```python
from build123d import *

# Parameters (mm, degrees)
SALIENTE_EXTRUIR1_DEPTH       = 3
REDONDEO1_R                   = 4
CROQUIS4_R                    = 2
CORTAR_EXTRUIR1_DEPTH         = 10
CROQUIS5_R                    = 2
CORTAR_EXTRUIR2_DEPTH         = 10
TALADRO_ROSCADO_M31_D         = 2.5
TALADRO_ROSCADO_M31_DEPTH     = 8.5
TALADRO_ROSCADO_M31_TIP       = 0.751075774
CROQUIS13_R                   = 2
CORTAR_EXTRUIR6_DEPTH         = 438.724799389
CROQUIS14_R                   = 2
CORTAR_EXTRUIR7_DEPTH         = 438.724799389
CORTAR_EXTRUIR9_DEPTH         = 438.724799389
TALADRO_ROSCADO_M32_D         = 2.5
TALADRO_ROSCADO_M32_DEPTH     = 8.5
TALADRO_ROSCADO_M32_TIP       = 0.751075774
TALADRO_ROSCADO_M33_OUTLINE_R = 1.25
TALADRO_ROSCADO_M33_DEPTH     = 3
CROQUIS22_R                   = 2
CORTAR_EXTRUIR10_DEPTH        = 438.724799389
CROQUIS23_R                   = 2
CORTAR_EXTRUIR11_DEPTH        = 438.724799389
TALADRO_ROSCADO_M34_OUTLINE_R = 1.25
TALADRO_ROSCADO_M34_DEPTH     = 3
CROQUIS26_R                   = 2
CORTAR_EXTRUIR12_DEPTH        = 438.724799389
TALADRO_ROSCADO_M35_OUTLINE_R = 1.25
TALADRO_ROSCADO_M35_DEPTH     = 3
CROQUIS31_R                   = 2
CORTAR_EXTRUIR13_DEPTH        = 438.724799389
CORTAR_EXTRUIR14_DEPTH        = 438.724799389


# Read off the part's stored shape, not the designer's step: Taladro roscado M33, Taladro roscado M34, Taladro roscado M35
with BuildPart() as part:
    # Croquis1 → Saliente-Extruir1 (new body)
    with BuildSketch(Plane(origin=(0, 0, 0), x_dir=(1, 0, 0), z_dir=(0, 1, 0))):
        Polygon((0, 0), (-413, 0), (-413, 45), (-338, 45), (-338, 123), (-190, 123), (-190, 107), (-125, 107), (-125, 145), (-75, 145), (-75, 97), (0, 97), align=None)
    saliente_extruir1 = extrude(amount=SALIENTE_EXTRUIR1_DEPTH)

    # Simetría1: Saliente-Extruir1 across plane
    add(saliente_extruir1.mirror(Plane(origin=(0, 3, 0), x_dir=(1, 0, 0), z_dir=(0, 0, -1))))

    # Redondeo1
    redondeo1_edges = [part.edges().sort_by_distance(p)[0] for p in [
        (-413, 1.5, -45),
        (-338, 1.5, -45),
        (-338, 1.5, -123),
        (-190, 1.5, -123),
        (-190, 1.5, -107),
        (-125, 1.5, -107),
        (-125, 1.5, -145),
        (-75, 1.5, -145),
        (-75, 1.5, -97),
        (0, 1.5, -97),
        (0, 1.5, 97),
        (-413, 1.5, 45),
        (-338, 1.5, 45),
        (-338, 1.5, 123),
        (-190, 1.5, 123),
        (-190, 1.5, 107),
        (-125, 1.5, 107),
        (-125, 1.5, 145),
        (-75, 1.5, 145),
        (-75, 1.5, 97),
    ]]
    fillet(redondeo1_edges, radius=REDONDEO1_R)

    # Croquis4 → Cortar-Extruir1 (cut)
    with BuildSketch(Plane(origin=(0, 3, 0), x_dir=(1, 0, 0), z_dir=(0, 1, 0))):
        with Locations(Location((-108.1, -50.5, 0), (0, 0, 270))):
            Circle(CROQUIS4_R)
    cortar_extruir1 = extrude(amount=-CORTAR_EXTRUIR1_DEPTH, mode=Mode.SUBTRACT)

    # Simetría2: Cortar-Extruir1 across plane
    add(cortar_extruir1.mirror(Plane.XY), mode=Mode.SUBTRACT)

    # Croquis5 → Cortar-Extruir2 (cut)
    with BuildSketch(Plane(origin=(0, 3, 0), x_dir=(1, 0, 0), z_dir=(0, 1, 0))):
        with Locations(Location((-288.1, -75, 0), (0, 0, 270))):
            Circle(CROQUIS5_R)
    cortar_extruir2 = extrude(amount=-CORTAR_EXTRUIR2_DEPTH, mode=Mode.SUBTRACT)

    # Simetría3: Cortar-Extruir2 across plane
    add(cortar_extruir2.mirror(Plane.XY), mode=Mode.SUBTRACT)

    # Taladro roscado M31
    with Locations(Plane(origin=(0, 3, 0), x_dir=(1, 0, 0), z_dir=(0, 1, 0))):
        with Locations((-329, 9.5), (-281.5, 9.5), (-281.5, -63), (-329, -63)):
            Hole(TALADRO_ROSCADO_M31_D / 2, depth=TALADRO_ROSCADO_M31_DEPTH)
            with Locations((0, 0, -(TALADRO_ROSCADO_M31_DEPTH + TALADRO_ROSCADO_M31_TIP / 2))):  # 118° drill point
                Cone(0, TALADRO_ROSCADO_M31_D / 2, TALADRO_ROSCADO_M31_TIP, mode=Mode.SUBTRACT)

    # Croquis13 → Cortar-Extruir6 (cut, through all)
    with BuildSketch(Plane(origin=(0, 3, 0), x_dir=(1, 0, 0), z_dir=(0, 1, 0))):
        with Locations(Location((-8, -90, 0), (0, 0, 270))):
            Circle(CROQUIS13_R)
    cortar_extruir6 = extrude(amount=-CORTAR_EXTRUIR6_DEPTH, mode=Mode.SUBTRACT)

    # Croquis14 → Cortar-Extruir7 (cut, through all)
    with BuildSketch(Plane(origin=(0, 3, 0), x_dir=(1, 0, 0), z_dir=(0, 1, 0))):
        with Locations(Location((-28, -90, 0), (0, 0, 270))):
            Circle(CROQUIS14_R)
    cortar_extruir7 = extrude(amount=-CORTAR_EXTRUIR7_DEPTH, mode=Mode.SUBTRACT)

    # Croquis16 → Cortar-Extruir9 (cut, through all)
    with BuildSketch(Plane(origin=(0, 3, 0), x_dir=(1, 0, 0), z_dir=(0, 1, 0))):
        with BuildLine():
            Line((-263.7, 41.75), (-249.7, 41.75))
            ThreePointArc((-249.7, 41.75), (-247.7, 43.75), (-249.7, 45.75))
            Line((-249.7, 45.75), (-263.7, 45.75))
            ThreePointArc((-263.7, 45.75), (-265.7, 43.75), (-263.7, 41.75))
        make_face()
        with BuildLine():
            Line((-263.7, -78.75), (-249.7, -78.75))
            ThreePointArc((-249.7, -78.75), (-247.7, -76.75), (-249.7, -74.75))
            Line((-249.7, -74.75), (-263.7, -74.75))
            ThreePointArc((-263.7, -74.75), (-265.7, -76.75), (-263.7, -78.75))
        make_face()
        with BuildLine():
            Line((-215.2, -43.75), (-201.2, -43.75))
            ThreePointArc((-201.2, -43.75), (-199.2, -41.75), (-201.2, -39.75))
            Line((-201.2, -39.75), (-215.2, -39.75))
            ThreePointArc((-215.2, -39.75), (-217.2, -41.75), (-215.2, -43.75))
        make_face()
        with BuildLine():
            Line((-144.61, -10.75), (-130.61, -10.75))
            ThreePointArc((-130.61, -10.75), (-128.61, -8.75), (-130.61, -6.75))
            Line((-130.61, -6.75), (-144.61, -6.75))
            ThreePointArc((-144.61, -6.75), (-146.61, -8.75), (-144.61, -10.75))
        make_face()
        with BuildLine():
            Line((-144.61, 39.75), (-130.61, 39.75))
            ThreePointArc((-130.61, 39.75), (-128.61, 41.75), (-130.61, 43.75))
            Line((-130.61, 43.75), (-144.61, 43.75))
            ThreePointArc((-144.61, 43.75), (-146.61, 41.75), (-144.61, 39.75))
        make_face()
        with BuildLine():
            Line((-193.11, 74.75), (-179.11, 74.75))
            ThreePointArc((-179.11, 74.75), (-177.11, 76.75), (-179.11, 78.75))
            Line((-179.11, 78.75), (-193.11, 78.75))
            ThreePointArc((-193.11, 78.75), (-195.11, 76.75), (-193.11, 74.75))
        make_face()
    extrude(amount=-CORTAR_EXTRUIR9_DEPTH, mode=Mode.SUBTRACT)

    # Taladro roscado M32
    with Locations(Plane(origin=(0, 3, 0), x_dir=(1, 0, 0), z_dir=(0, 1, 0))):
        with Locations((-315, 34), (-315, 109)):
            Hole(TALADRO_ROSCADO_M32_D / 2, depth=TALADRO_ROSCADO_M32_DEPTH)
            with Locations((0, 0, -(TALADRO_ROSCADO_M32_DEPTH + TALADRO_ROSCADO_M32_TIP / 2))):  # 118° drill point
                Cone(0, TALADRO_ROSCADO_M32_D / 2, TALADRO_ROSCADO_M32_TIP, mode=Mode.SUBTRACT)

    # Taladro roscado M33 outline → Taladro roscado M33 (cut)
    with BuildSketch(Plane(origin=(0, 0, 0), x_dir=(1, 0, 0), z_dir=(0, 1, 0))):
        with Locations((-250, 86)):
            Circle(TALADRO_ROSCADO_M33_OUTLINE_R)
        with Locations((-274, 86)):
            Circle(TALADRO_ROSCADO_M33_OUTLINE_R)
    extrude(amount=TALADRO_ROSCADO_M33_DEPTH, mode=Mode.SUBTRACT)

    # Croquis22 → Cortar-Extruir10 (cut, through all)
    with BuildSketch(Plane(origin=(0, 3, 0), x_dir=(1, 0, 0), z_dir=(0, 1, 0))):
        with Locations(Location((-247.2, 67.5, 0), (0, 0, 270))):
            Circle(CROQUIS22_R)
        with Locations(Location((-217.2, 67.5, 0), (0, 0, 270))):
            Circle(CROQUIS22_R)
        with Locations(Location((-217.2, -100.5, 0), (0, 0, 270))):
            Circle(CROQUIS22_R)
        with Locations(Location((-247.2, -100.5, 0), (0, 0, 270))):
            Circle(CROQUIS22_R)
    extrude(amount=-CORTAR_EXTRUIR10_DEPTH, mode=Mode.SUBTRACT)

    # Croquis23 → Cortar-Extruir11 (cut, through all)
    with BuildSketch(Plane(origin=(0, 3, 0), x_dir=(1, 0, 0), z_dir=(0, 1, 0))):
        with Locations(Location((-176.61, 100.5, 0), (0, 0, 270))):
            Circle(CROQUIS23_R)
        with Locations(Location((-146.61, 100.5, 0), (0, 0, 270))):
            Circle(CROQUIS23_R)
        with Locations(Location((-146.61, -67.5, 0), (0, 0, 270))):
            Circle(CROQUIS23_R)
        with Locations(Location((-176.61, -67.5, 0), (0, 0, 270))):
            Circle(CROQUIS23_R)
    extrude(amount=-CORTAR_EXTRUIR11_DEPTH, mode=Mode.SUBTRACT)

    # Taladro roscado M34 outline → Taladro roscado M34 (cut)
    with BuildSketch(Plane(origin=(0, 0, 0), x_dir=(1, 0, 0), z_dir=(0, 1, 0))):
        with Locations((-118, -27)):
            Circle(TALADRO_ROSCADO_M34_OUTLINE_R)
        with Locations((-118, -3)):
            Circle(TALADRO_ROSCADO_M34_OUTLINE_R)
    extrude(amount=TALADRO_ROSCADO_M34_DEPTH, mode=Mode.SUBTRACT)

    # Croquis26 → Cortar-Extruir12 (cut, through all)
    with BuildSketch(Plane(origin=(0, 3, 0), x_dir=(1, 0, 0), z_dir=(0, 1, 0))):
        with Locations(Location((-118.122816505, -114, 0), (0, 0, 270))):
            Circle(CROQUIS26_R)
        with Locations(Location((-82.122816505, -114, 0), (0, 0, 270))):
            Circle(CROQUIS26_R)
        with Locations(Location((-82.122816505, -128, 0), (0, 0, 270))):
            Circle(CROQUIS26_R)
        with Locations(Location((-118.122816505, -128, 0), (0, 0, 270))):
            Circle(CROQUIS26_R)
    cortar_extruir12 = extrude(amount=-CORTAR_EXTRUIR12_DEPTH, mode=Mode.SUBTRACT)

    # Simetría4: Cortar-Extruir12 across plane
    add(cortar_extruir12.mirror(Plane.XY), mode=Mode.SUBTRACT)

    # Taladro roscado M35 outline → Taladro roscado M35 (cut)
    with BuildSketch(Plane(origin=(0, 0, 0), x_dir=(1, 0, 0), z_dir=(0, 1, 0))):
        with Locations((-5.5, 0)):
            Circle(TALADRO_ROSCADO_M35_OUTLINE_R)
        with Locations((-5.5, -45)):
            Circle(TALADRO_ROSCADO_M35_OUTLINE_R)
        with Locations((-80.5, 0)):
            Circle(TALADRO_ROSCADO_M35_OUTLINE_R)
        with Locations((-80.5, 45)):
            Circle(TALADRO_ROSCADO_M35_OUTLINE_R)
    extrude(amount=TALADRO_ROSCADO_M35_DEPTH, mode=Mode.SUBTRACT)

    # Simetría5: Cortar-Extruir6, Cortar-Extruir7 across plane
    add(cortar_extruir6.mirror(Plane.XY), mode=Mode.SUBTRACT)
    add(cortar_extruir7.mirror(Plane.XY), mode=Mode.SUBTRACT)

    # Croquis31 → Cortar-Extruir13 (cut, through all)
    with BuildSketch(Plane(origin=(0, 3, 0), x_dir=(1, 0, 0), z_dir=(0, 1, 0))):
        with Locations(Location((-403.7, 20, 0), (0, 0, 270))):
            Circle(CROQUIS31_R)
        with Locations(Location((-374.7, 20, 0), (0, 0, 270))):
            Circle(CROQUIS31_R)
    cortar_extruir13 = extrude(amount=-CORTAR_EXTRUIR13_DEPTH, mode=Mode.SUBTRACT)

    # Simetría6: Cortar-Extruir13 across plane
    add(cortar_extruir13.mirror(Plane.XY), mode=Mode.SUBTRACT)

    # Croquis32 → Cortar-Extruir14 (cut, through all)
    with BuildSketch(Plane.XZ):
        with BuildLine():
            Line((-185.11, 41.75), (-193.11, 41.75))
            ThreePointArc((-193.11, 41.75), (-195.11, 43.75), (-193.11, 45.75))
            Line((-193.11, 45.75), (-185.11, 45.75))
            Line((-185.11, 45.75), (-179.11, 45.75))
            ThreePointArc((-179.11, 45.75), (-177.11, 43.75), (-179.11, 41.75))
            Line((-179.11, 41.75), (-185.11, 41.75))
        make_face()
        with BuildLine():
            Line((-207.2, -10.75), (-215.2, -10.75))
            ThreePointArc((-215.2, -10.75), (-217.2, -8.75), (-215.2, -6.75))
            Line((-215.2, -6.75), (-207.2, -6.75))
            Line((-207.2, -6.75), (-201.2, -6.75))
            ThreePointArc((-201.2, -6.75), (-199.2, -8.75), (-201.2, -10.75))
            Line((-201.2, -10.75), (-207.2, -10.75))
        make_face()
    extrude(amount=-CORTAR_EXTRUIR14_DEPTH, mode=Mode.SUBTRACT)


solid = part.part
```
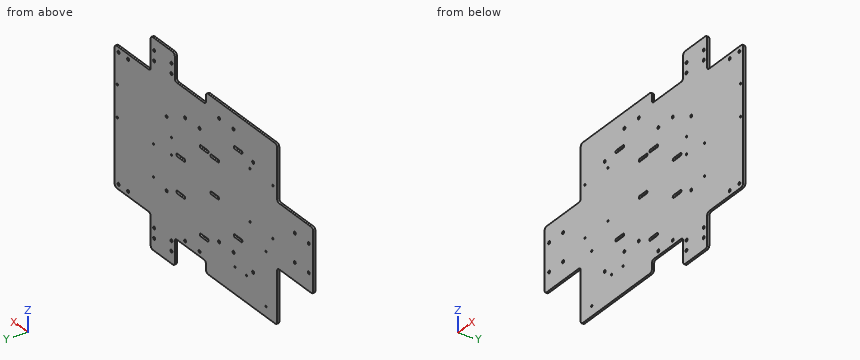
The listing builds one solid part. Answer for the finished solid, in the listing's coordinates (mm). Round coordinates to 2 decimals unless told otherwise and drop trailing zeros. Loops run counter-clockwise (first coordinate to the right, second up) from the corner with the lowest first, then second, coordinate; pieces in that order, holes last. Notation, with made-up numbers: (-9, -37.75) - (25, -37.75) arc R25 ccw to (25, -21.75) - close; hole circle Ø10 at (33, 71.25). An arc over 180 degrees is marked (long way). Use one line per item in the form item = value. Start each with the question number.
1. The part is cut by section A-A on z = 57.5. Determine the outline of the cut face in (x, y), then the cut area to 3 significant figures.
2. Consider line 1 (X direction, y = 2.05, z = 128); line 2 (Z direction, x = -5.5, y = 1.6); line 3 (Z direction, x = -176.61, y = 2.25). Determine where each line is inside the solid, lowest interval first. Write a range as [from, to].
3. Given pin 1 Ø1.5 at (x, y) = (-254, 1) entering from -Z; pin 2 Ø1 at (y, z) = (0.5, 52.5) entering from -X; pin 3 Ø0.9 at (y, z) = (1, 113.5) entering from +X, each flat-ended and moving along its own axis, determine where each tip first touches the part or whether it passes through.
4. The part is cut by section B-B on y = 0.45. Give the number of separate pieces and of enclosed holes in the cut face, then the cut area to 3 significant figures.
Geometry check:
q1.outline = (-338, 0) - (0, 0) - (0, 3) - (-338, 3) - close
q1.area = 1,010 mm^2
q2.line_1 = [-125, -120.12], [-116.12, -84.12], [-80.12, -75]
q2.line_2 = [-97, -1.25], [1.25, 43.75], [46.25, 97]
q2.line_3 = [-107, -102.5], [-98.5, 65.5], [69.5, 107]
q3.pin_1 = -123
q3.pin_2 = -338
q3.pin_3 = -75
q4.separate_pieces = 1
q4.enclosed_holes = 50
q4.area = 85,100 mm^2
